Input: dimensioned drawing with shaded views. Units: mm. Origin: part minimum x, y, z. Round coordinates to 2 decimals unless told otherwise and drop trailing zeros. Order: outer loops, then holes, each group sorted by start corner. A loop starts at its lowest first (then second) coordinate and runs counter-clockwise, first axis right, second up.
Item 1: First-contact query: pin 1 (1.5 mm diameter, centred on x = 1.5, z = 1, fed in from -Y); pin 2 (1 mm diameter, centred on y = 162.5, z = 13, fed in from -X); pin 3 (1.5 mm diameter, centred on x = 1.5, z = 1.5, fed in from +Y); pin 4 (1.5 mm diameter, centred on x = 2, y = 198, fed in from -Z). Flat tips, straight axial feed; report the tip coordinate or a pass-through.
Item 2: Line query: L1, parallel to Y at x = 0.8, z = 2.25; L2, parallel to Y at x = 2.6, z = 13.25. Output: solid intervals per line, ascending.
Item 3: Cut plane A-A on x = 1.75. Output: boundary loops of the cut face in (y, z), then the cut area to 3 significant figures.
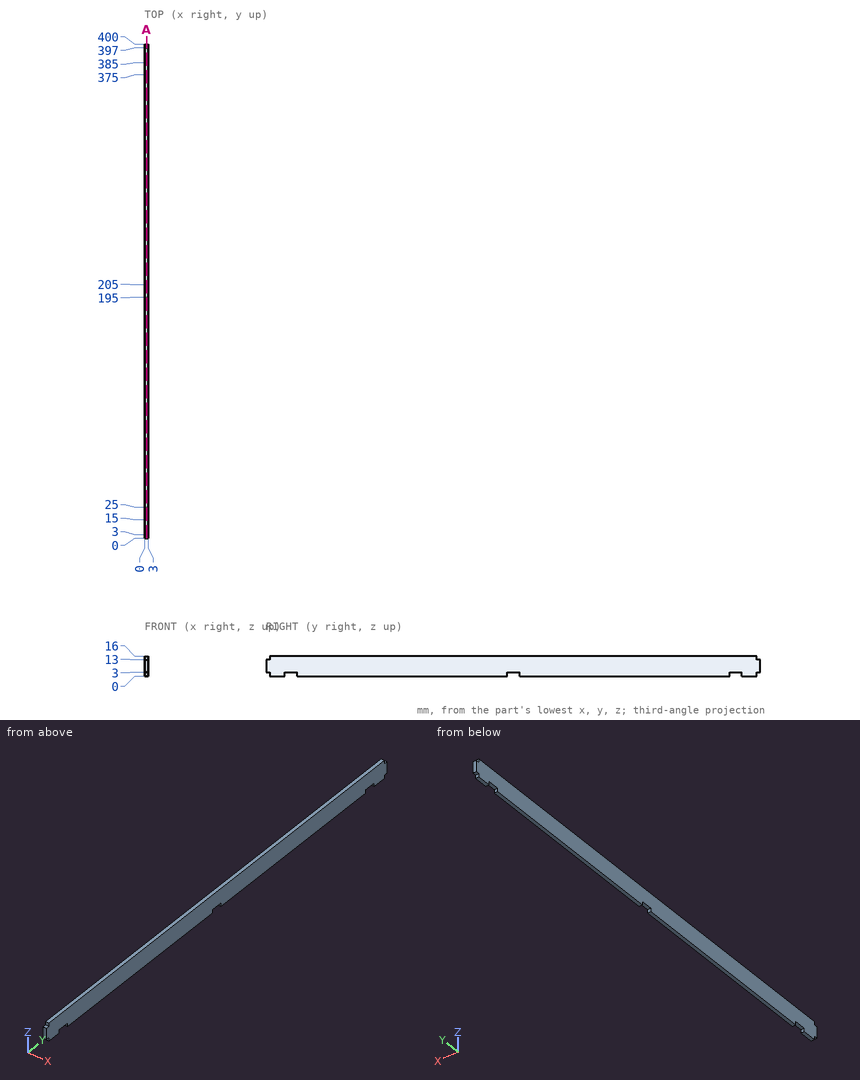
From the geometry:
1. pin 1: stops at y = 3
1. pin 2: stops at x = 0
1. pin 3: stops at y = 397
1. pin 4: stops at z = 3
2. L1: y = 3 to 15, 25 to 195, 205 to 375, 385 to 397
2. L2: y = 3 to 397
3. outline: (0, 3) - (3, 3) - (3, 0) - (15, 0) - (15, 3) - (25, 3) - (25, 0) - (195, 0) - (195, 3) - (205, 3) - (205, 0) - (375, 0) - (375, 3) - (385, 3) - (385, 0) - (397, 0) - (397, 3) - (400, 3) - (400, 13) - (397, 13) - (397, 16) - (3, 16) - (3, 13) - (0, 13) - close
3. area: 6,270 mm2
